Part model, mm, in its own coordinate system. A direction names the side the tool comes from. Round coordinates to 2 decimals unless told otherwise and drop trailing zeros. Loops run counter-clockwise (first coordinate to the right, second up) from the corner with the lowest first, then second, coordinate; pieces in that order, holes last.
(1) Cut at D-D on x = 7.5. List the corners of the cut face in (y, z).
(2) Cut at A-A on y = 16. List the corners of the cut face in (x, z), then the cut area to 3 significant figures.
(3) Cut at C-C on x = 40.5. List the corners of the cut face in (y, z), then the cut area to 3 significant figures.
(4) Cut at B-B on z = 13.75. List the corners of the cut face in (x, y), then the cut area to 3 significant figures.
(5) Probe probe 1 along X at (y, z) = (47, 4.25); probe 2 along Y at (x, z) = (27, 25.25); probe 3 along X at (y, z) = (34, 16.25). List the from-to ranges inside material, lowest first.
(6) Mould opens along Y. For faces 4 (the face through (38, 38, 10)), 5 (the face through (0, 37, 11)), 6 (the face through (38, 16, 14)) say: +Y half, -Y half, draft (parallel to the pull), parting line (faces both ways), or undercut.
(7) Tool access for faces 1 (the face through (26, 50, 10)), 2 (the face through (17, 48, 20)), 3 (the face through (60, 15, 14)): list every direction of +Z, -Z, +X, -X, +Y, -Y with a clear straight run to the whole face (end or side of a thin tool).
(8) Flat gauge pins, fed straight in: pin 1 (3.5 mm diameter, centred on y = 41, z = 14.5, fed in from +X); pin 2 (3.5 mm diameter, centred on x = 27.5, z = 9.5, fed in from +Y); pin 3 (10 mm diameter, centred on y = 57, z = 18, fed in from +X). Where does each tip first touch, or does it go through?
from build123d import *

# Parameters (mm, degrees)
SKETCH1_W           = 60
SKETCH1_H           = 30
SKETCH1_R           = 6
BOSS_EXTRUDE1_DEPTH = 28
BOSS_EXTRUDE2_DEPTH = 20


with BuildPart() as part:
    # Sketch1 → Boss-Extrude1 (new body)
    with BuildSketch(Plane.XY):
        with Locations((30, 15)):
            Rectangle(SKETCH1_W, SKETCH1_H)
        with Locations((44, 16)):
            Circle(SKETCH1_R, mode=Mode.SUBTRACT)
    extrude(amount=BOSS_EXTRUDE1_DEPTH)

    # Sketch3 → Boss-Extrude2 (add)
    with BuildSketch(Plane.XY):
        Polygon((0, 30), (0, 75), (20, 75), (20, 50), (32, 50), (32, 38), (44, 38), (44, 30), align=None)
    extrude(amount=BOSS_EXTRUDE2_DEPTH)


solid = part.part
Final values:
1. outline: (0, 0) - (75, 0) - (75, 20) - (30, 20) - (30, 28) - (0, 28) - close
2. outline: (0, 0) - (38, 0) - (38, 28) - (0, 28) - close; (50, 0) - (60, 0) - (60, 28) - (50, 28) - close
2. area: 1,340 mm2
3. outline: (0, 0) - (11.13, 0) - (11.13, 28) - (0, 28) - close; (20.87, 0) - (38, 0) - (38, 20) - (30, 20) - (30, 28) - (20.87, 28) - close
3. area: 727 mm2
4. outline: (0, 0) - (60, 0) - (60, 30) - (44, 30) - (44, 38) - (32, 38) - (32, 50) - (20, 50) - (20, 75) - (0, 75) - close; hole circle Ø12 at (44, 16)
4. area: 2,920 mm2
5. probe 1: x = 0 to 32
5. probe 2: y = 0 to 30
5. probe 3: x = 0 to 44
6. face 4: +Y half
6. face 5: draft
6. face 6: undercut
7. face 1: +Z, -Z, +X, +Y
7. face 2: +Z, +X, -X, +Y
7. face 3: +Z, -Z, +X, +Y, -Y
8. pin 1: stops at x = 32
8. pin 2: stops at y = 50
8. pin 3: stops at x = 20
